Work out the finished part from the listing and answer in its coordinate system (mm). Face numbers are marked on the shaded views. A direction names the side the tool comes from. Round coordinates to 2 decimals unless told otherwise and drop trailing zeros. Loops run counter-clockwise (first coordinate to the right, second up) from the corner with the lowest first, then second, coordinate; pieces in that order, holes last. Notation, with made-up numbers: (22, -17.5) - (57, -17.5) arc R23 cw to (57, -7.5) - close; hole circle Ø5 at (7.5, 7). An arc over 180 degrees is marked (long way). Return JSON: item names as keys, results as strings.
Autodesk Inventor part; units mm, degrees
ref_plane "YZ Plane" through (0, 0, 0) normal (1, 0, 0) x (0, 1, 0)
ref_plane "XZ Plane" through (0, 0, 0) normal (0, 1, 0) x (-1, 0, 0)
ref_plane "XY Plane" through (0, 0, 0) normal (0, 0, 1) x (1, 0, 0)
sketch "Sketch1" plane through (0, 0, 0) normal (0, 0, 1) x (1, 0, 0)
  circle A0 centre (0, 0) radius 6.1
  line L0 (-12.5, -10) -> (12.5, -10)
  line L1 (12.5, -10) -> (12.5, 10)
  line L2 (12.5, 10) -> (-12.5, 10)
  line L3 (-12.5, 10) -> (-12.5, -10)
  line L4 (-12.5, -10) -> (12.5, 10) construction
  line L5 (12.5, -10) -> (-12.5, 10) construction
  dimension "d0" = 12.2
  dimension "d1" = 25
  dimension "d2" = 20
extrude "Extrusion1" add sketch "Sketch1" along normal blind 20
sketch "Sketch2" plane through (-12.5, 10, 0) normal (0, 1, 0) x (1, 0, 0)
  line L0 (0, 0) -> (0, -20) construction
  line L1 (25, -20) -> (0, -20) construction
  line L2 (0, 0) -> (25, -20) construction
  line L3 (0, -20) -> (25, 0) construction
  circle A0 centre (12.5, -10) radius 0.95
  point P0 (12.5, 0)
  dimension "d5" = 1.9
extrude "Extrusion2" cut sketch "Sketch2" against normal blind 100
sketch "Sketch3" plane through (-12.5, 10, 0) normal (0, 1, 0) x (1, 0, 0)
  circle A0 centre (12.5, -10) radius 0.95
  line L0 (25, 0) -> (0, 0)
  line L1 (0, 0) -> (0, -20)
  line L2 (25, -20) -> (0, -20)
  line L3 (25, 0) -> (25, -20)
  circle A1 centre (12.5, -10) radius 7.5
  point P0 (12.5, 0)
  dimension "d8" = 15
extrude "Extrusion3" add sketch "Sketch3" along normal blind 15 contours A1
sketch "Sketch4" plane through (-12.5, -10, 0) normal (0, -1, 0) x (1, 0, 0)
  line L0 (32.5, 25) -> (-7.5, 25)
  line L1 (-7.5, 25) -> (-7.5, -5)
  line L2 (-7.5, -5) -> (32.5, -5)
  line L3 (32.5, -5) -> (32.5, 25)
  circle A0 centre (12.5, 10) radius 0.95
  line L4 (32.5, 25) -> (-7.5, -5) construction
  line L5 (-7.5, 25) -> (32.5, -5) construction
  point P0 (12.5, 0)
  dimension "d11" = 30
  dimension "d12" = 40
extrude "Extrusion4" add sketch "Sketch4" along normal blind 3
sketch "Sketch6" plane through (20, -10, -5) normal (0, 0, -1) x (-1, 0, 0)
  line L0 (-13.3468, 43.0165) -> (63.7046, 43.0165)
  line L1 (63.7046, 43.0165) -> (63.7046, -16.6019)
  line L2 (63.7046, -16.6019) -> (-13.3468, -16.6019)
  line L3 (-13.3468, -16.6019) -> (-13.3468, 43.0165)
  point P0 (20, 10)
extrude "Extrusion6" cut sketch "Sketch6" against normal blind 10
sketch "Sketch8" plane through (-12.5, 25, 0) normal (0, 1, 0) x (1, 0, 0)
  circle A0 centre (12.5, -10) radius 0.95
  point P0 (12.5, 0)
extrude "Extrusion8" cut sketch "Sketch8" against normal blind 100
sketch "Sketch9" plane through (0, 0, 20) normal (0, 0, 1) x (1, 0, 0)
  line L0 (-2, 5.7628) -> (-2, 3)
  line L1 (-2, 3) -> (2, 3)
  line L2 (2, 3) -> (2, 5.7628)
  circle A0 centre (0, 0) radius 6.1
  line L3 (12.5, -10) -> (12.5, 10)
  line L4 (12.5, 10) -> (-12.5, 10)
  line L5 (-12.5, 10) -> (-12.5, -10)
  line L6 (-12.5, -10) -> (12.5, -10)
  circle A1 centre (0, 0) radius 6.1
  dimension "d28" = 2
  dimension "d29" = 2
  dimension "d30" = 3
extrude "Extrusion9" add sketch "Sketch9" against normal blind 5 contours L0 L1 L2 A0 picked at (0.2259, -0.0207)
sketch "Sketch10" plane through (0, 0, 15) normal (0, 0, -1) x (-1, 0, 0)
  circle A0 centre (0, 0) radius 4.9
  dimension "d33" = 9.8
extrude "Extrusion10" add sketch "Sketch10" along normal blind 15
sketch "Sketch11" plane through (-12.5, 25, 0) normal (0, 1, 0) x (1, 0, 0)
  circle A0 centre (12.5, -10) radius 0.95
  point P0 (12.5, 0)
extrude "Extrusion11" cut sketch "Sketch11" against normal blind 100
properties part number "Feather_0_template"
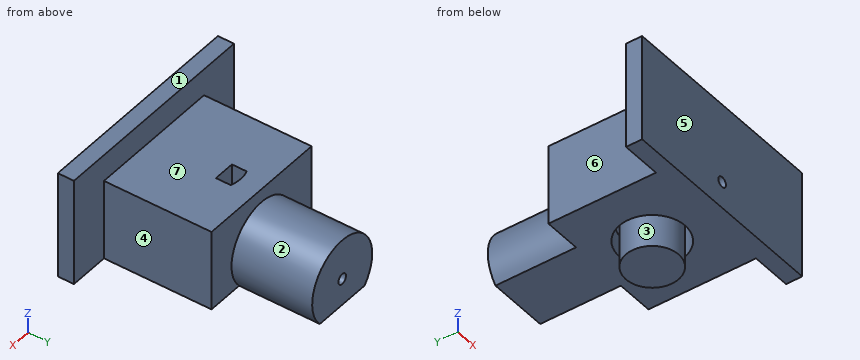
1) Find the intervals of material crossed by L1, parallel to Y at x = 0, z = 14.75; L2, parallel to X at y = 0, z = 10; L3, parallel to Z at x = 0, y = -0.5, in increasing order.
Verdict:
{"L1": "y = -13 to -6.1, -4.9 to 4.9, 6.1 to 25", "L2": "x = -12.5 to -6.1, -4.9 to -0.95, 0.95 to 4.9, 6.1 to 12.5", "L3": "z = 0 to 9.05, 10.95 to 20"}
2) Section D-D (z = 10) is taken. Give the vertices of the cut face in (x, y).
Verdict:
{"outline": "(-20, -13) - (-0.95, -13) - (-0.95, -6.03) arc R6.1 cw to (-0.95, 6.03) - (-0.95, 25) - (-7.5, 25) - (-7.5, 10) - (-12.5, 10) - (-12.5, -10) - (-20, -10) - close; (-0.95, -4.81) - (-0.95, 4.81) arc R4.9 ccw to start; (0.95, -13) - (20, -13) - (20, -10) - (12.5, -10) - (12.5, 10) - (7.5, 10) - (7.5, 25) - (0.95, 25) - (0.95, 6.03) arc R6.1 cw to (0.95, -6.03) - close; (0.95, -4.81) arc R4.9 ccw to (0.95, 4.81) - close"}
3) Section A-A (z = 6.5) is taken. Give the vertices of the cut face in (x, y), and give its area (3 significant figures).
Verdict:
{"outline": "(-20, -13) - (20, -13) - (20, -10) - (12.5, -10) - (12.5, 10) - (6.63, 10) - (6.63, 25) - (-6.63, 25) - (-6.63, 10) - (-12.5, 10) - (-12.5, -10) - (-20, -10) - close; circle Ø9.8 at (0, 0); hole circle Ø12.2 at (0, 0)", "area": "778 mm2"}
4) Flat-ended cylindrical pins translate along their axes: pin 1 (6 mm diameter, centred on y = 15, z = 6, fed in from +X); pin 2 (8 mm diameter, centred on x = 10.5, y = 0.5, fed in from -Z); pin 3 (4.5 mm diameter, centred on y = 2.5, z = 13, fed in from +X). Find the tip coordinate at first contact, or state that the pin passes through.
Verdict:
{"pin 1": "stops at x = 7.43", "pin 2": "stops at z = 5", "pin 3": "stops at x = 12.5"}
5) Section C-C (y = 0) is taken. Give the vertices of the cut face in (x, z), and give its area (3 significant figures).
Verdict:
{"outline": "(-12.5, 5) - (-6.1, 5) - (-6.1, 15) - (-4.9, 15) - (-4.9, 0) - (4.9, 0) - (4.9, 15) - (6.1, 15) - (6.1, 5) - (12.5, 5) - (12.5, 20) - (-12.5, 20) - close; hole circle Ø1.9 at (0, 10)", "area": "397 mm2"}
6) Section B-B (x = 0) is taken. Count the separate pieces of the cut face and the enclosed holes in it, and give its area (3 significant figures).
Verdict:
{"separate pieces": "5", "enclosed holes": "0", "area": "489 mm2"}
7) Determine the mould class of the marked faces 1, 2 and 3 for opening direction X: pulls with the +X half, pulls with the -X half, needs draft (parallel to the pull), parting line crosses it, or undercut.
Verdict:
{"face 1": "needs draft", "face 2": "parting line crosses it", "face 3": "undercut"}
8) A tool of negligible diameter and unlimited length cuts with its end or side. For the marked faces 4, 5, 6 and 7, from which of +Z, -Z, +X, -X, +Y, -Y can it reach the whole face along a straight path? Write none if from no direction.
Verdict:
{"face 4": "+Z, -Z, +X, +Y", "face 5": "+Z, -Z, +X, -X, -Y", "face 6": "+Z, -Z, -X, +Y", "face 7": "+Z, +X, -X, +Y"}
